Job drawing, mm, ordinate dimensions from the low corner. One solid piece. A direction names the side the tool comes from. Give positions to 0.01 mm unless a question says otherwise; leave off trailing zeros. Order: outer loops, then holes, each group sorted by start corner. A loop starts at its lowest first (then second) coordinate and runs counter-clockwise, first axis right, second up.
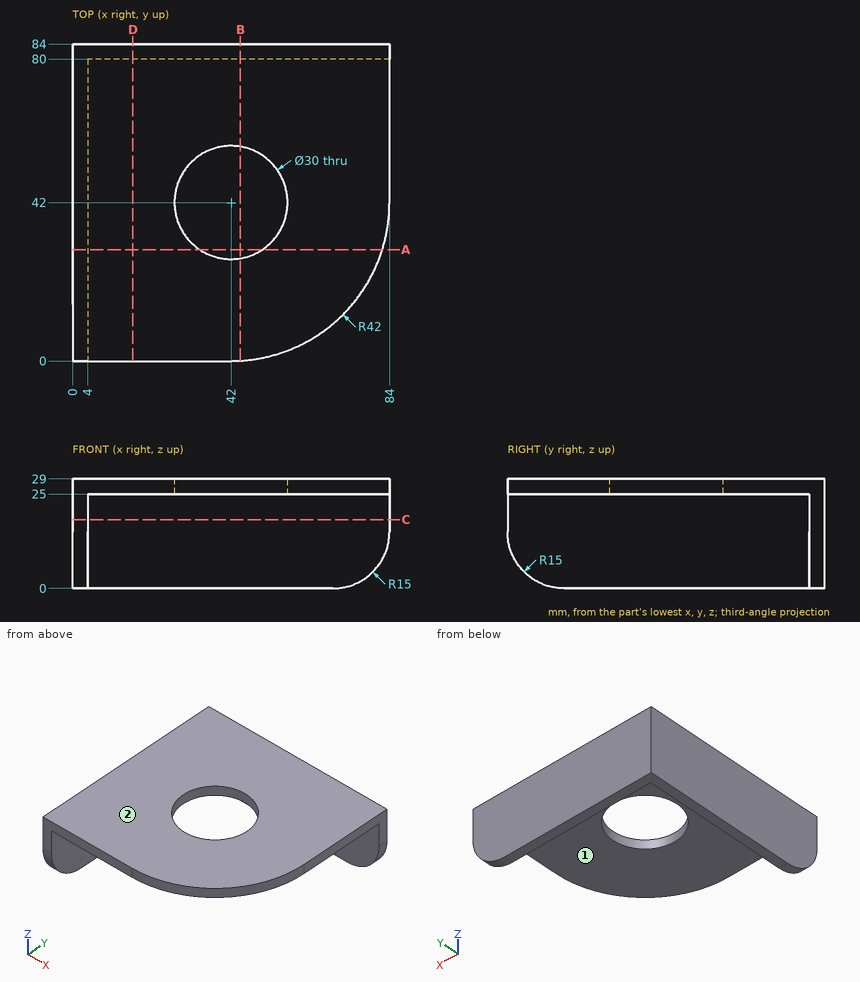
Item 1: Drill centre lines: probe 1 along Y at (x, z) = (42, 27.05); probe 2 along Y at (x, z) = (62.5, 9.25); probe 3 along X at (y, z) = (19, 19). Where is each one in solid material? Low to high.
Item 2: Band-saw the part on C-C on z = 18.25. List the corners of the cut face in (x, y).
Item 3: Which spindle directions (+Z, -Z, +X, -X, +Y, -Y) get a long thin tool onto all of the face, cutting with end or side? Do the marked faces 1 and 2. Say none if no direction does.
Item 4: Band-saw the part on B-B on x = 44.5. List the corners of the cut face in (y, z), plus the area to 3 significant figures.
Item 5: Band-saw the part on A-A on y = 29.5. List the corners of the cut face in (x, z), plus the area to 3 significant figures.
Item 6: Drop flat-ended pins along their axis: P1, Ø18, axis at x = 42, y = 42, coming from the +Z side; P2, Ø4, axis at y = 38.5, z = 13, coming from the +X side; P3, Ø1, axis at x = 61.5, z = 21, coming from the -Y side; P4, Ø2, axis at x = 58, y = 71, coming from the -Z side. Give the stop position or say it passes through.
Item 7: Band-saw the part on D-D on x = 16. List the corners of the cut face in (y, z), plus the area to 3 significant figures.
Working result:
1. probe 1: y = 0 to 27, 57 to 84
1. probe 2: y = 80 to 84
1. probe 3: x = 0 to 4
2. outline: (0, 0) - (4, 0) - (4, 80) - (84, 80) - (84, 84) - (0, 84) - close
3. face 1: -Z, +X, -Y
3. face 2: +Z, +X, -X, +Y, -Y
4. outline: (0.07, 25) - (27.21, 25) - (27.21, 29) - (0.07, 29) - close; (56.79, 25) - (80, 25) - (80, 0) - (84, 0) - (84, 29) - (56.79, 29) - close
4. area: 317 mm2
5. outline: (0, 0) - (4, 0) - (4, 25) - (33.71, 25) - (33.71, 29) - (0, 29) - close; (50.29, 25) - (82.1, 25) - (82.1, 29) - (50.29, 29) - close
5. area: 362 mm2
6. P1: passes through
6. P2: stops at x = 4
6. P3: stops at y = 80
6. P4: stops at z = 25
7. outline: (0, 25) - (80, 25) - (80, 0) - (84, 0) - (84, 29) - (0, 29) - close
7. area: 436 mm2
